```python
from build123d import *

# Parameters (mm, degrees)
SKETCH_1_W          = 18
SKETCH_1_H          = 29
SKETCH_1_R          = 1.75
EXTRUDE_1_DEPTH     = 19
SKETCH_2_R          = 4
CUT_EXTRUDE_1_DEPTH = 20
FILLET_1_R          = 2


with BuildPart() as part:
    # 草图1 → 凸台-拉伸1 (new body)
    with BuildSketch(Plane(origin=(0, 0, 0), x_dir=(1, 0, 0), z_dir=(0, 1, 0))):
        with Locations((0, 24.5)):
            Rectangle(SKETCH_1_W, SKETCH_1_H)
        with Locations(Location((6, 15, 0), (0, 0, 270))):
            Circle(SKETCH_1_R, mode=Mode.SUBTRACT)
        with Locations(Location((6, 35, 0), (0, 0, 270))):
            Circle(SKETCH_1_R, mode=Mode.SUBTRACT)
    extrude(amount=EXTRUDE_1_DEPTH)

    # 草图2 → 切除-拉伸1 (cut)
    with BuildSketch(Plane.ZY.offset(9)):
        with Locations((-25, 11)):
            Circle(SKETCH_2_R)
        with Locations((-5, 11)):
            Circle(SKETCH_2_R)
    extrude(amount=-CUT_EXTRUDE_1_DEPTH, mode=Mode.SUBTRACT)

    # 圆角1
    fillet_1_edges = [part.edges().sort_by_distance(p)[0] for p in [
        (0, 19, -10),
        (0, 0, -10),
        (0, 0, -39),
        (0, 19, -39),
    ]]
    fillet(fillet_1_edges, radius=FILLET_1_R)


solid = part.part
```
Design review of the part built by this model. Coordinates are the model's own, in mm. Round coordinates to 2 decimals unless told otherwise and drop trailing zeros. Write each loop counter-clockwise with the first axis right and the second up, starting at its lowest first coordinate (ties: lowest second). Pieces come first, ordered by that corner, then holes. Notation, with made-up numbers: (68.25, -28) -> (102.25, -28) arc R31 cw to (102.25, -3) -> close; hole circle Ø3 at (-3, 78). An arc over 180 degrees is marked (long way). Answer in a Markdown table with one row per item.
Q1. Take a section at D-D, the plane x = 4.75. State the section outline as (y, z) points, then the cut area to 3 significant figures.
The answers:
| item | result |
|---|---|
| outline | (0, -37) arc R2 ccw to (2, -39) -> (17, -39) arc R2 ccw to (19, -37) -> (19, -36.22) -> (0, -36.22) -> close; (0, -33.78) -> (19, -33.78) -> (19, -16.22) -> (0, -16.22) -> close; (0, -13.78) -> (19, -13.78) -> (19, -12) arc R2 ccw to (17, -10) -> (2, -10) arc R2 ccw to (0, -12) -> close; hole circle Ø8 at (11, -25) |
| area | 404 mm² |
Q2. Take a section at B-B, the plane y = 13. State the section outline as (x, z) points, then the cut area to 3 significant figures.
The answers:
| item | result |
|---|---|
| outline | (-9, -39) -> (9, -39) -> (9, -28.46) -> (-9, -28.46) -> close; (-9, -21.54) -> (9, -21.54) -> (9, -10) -> (-9, -10) -> close; hole circle Ø3.5 at (6, -35); hole circle Ø3.5 at (6, -15) |
| area | 378 mm² |
Q3. To check wall thickness, follow L1, parallel to Y at x = -2.75, z = -25; L2, parallel to Z at x = 7.25, y = 6.25; L3, parallel to X at y = 13, z = -15. State the ranges of each line that lie inside material, in increasing order. Write a range as [from, to].
The answers:
| item | result |
|---|---|
| L1 | [0, 7], [15, 19] |
| L2 | [-39, -36.22], [-33.78, -16.22], [-13.78, -10] |
| L3 | [-9, 4.25], [7.75, 9] |
Q4. Take a section at C-C, the plane x = -5. State the section outline as (y, z) points, then the cut area to 3 significant figures.
The answers:
| item | result |
|---|---|
| outline | (0, -37) arc R2 ccw to (2, -39) -> (17, -39) arc R2 ccw to (19, -37) -> (19, -12) arc R2 ccw to (17, -10) -> (2, -10) arc R2 ccw to (0, -12) -> close; hole circle Ø8 at (11, -25) |
| area | 497 mm² |
Q5. Take a section at A-A, the plane z = -35. State the section outline as (x, y) points, then the cut area to 4 significant figures.
The answers:
| item | result |
|---|---|
| outline | (-9, 0) -> (4.25, 0) -> (4.25, 19) -> (-9, 19) -> close; (7.75, 0) -> (9, 0) -> (9, 19) -> (7.75, 19) -> close |
| area | 275.5 mm² |
Q6. Clearance check with flat-ended pins moving along their axes: pin 1 Ø3 at (x, z) = (6, -16) entering from +Y; pin 2 Ø2 at (x, z) = (6, -35) entering from +Y. State where each tip first meets the part, or that it passes through.
The answers:
| item | result |
|---|---|
| pin 1 | y = 19 |
| pin 2 | through |
Q7. Draft analysis for pull direction Z (two halves, no side actions). For faces 1 (the face through (0, 19, -25)), 2 (the face through (0, 9, -10)), 3 (the face through (0.13, 0.57, -38.4)), 4 (the face through (4.94, 9.37, -36.39)), state which applies: +Z half, -Z half, draft (parallel to the pull), parting line (faces both ways), or undercut.
The answers:
| item | result |
|---|---|
| face 1 | draft |
| face 2 | +Z half |
| face 3 | -Z half |
| face 4 | undercut |
